Geometry check sheet. Reference: the model listing, model coordinates, mm. Face numbers are marked on the shaded views. A direction names the side the tool comes from. Coordinates: 2 decimals unless noted, no trailing zeros. Order: outer loops, then holes, each group sorted by start corner. A loop starts at its lowest first (then second) coordinate and runs counter-clockwise, first axis right, second up.
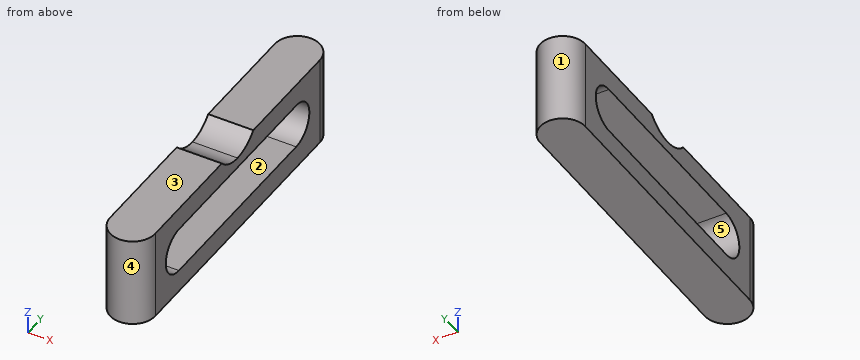
```python
from build123d import *

# Parameters (mm, degrees)
F1_DEPTH = 25.4
F3_DEPTH = 25.4
F5_DEPTH = 25.4


with BuildPart() as f1:
    # F0 (on Top) → F1 (new body)
    with BuildSketch(Plane.XY):
        with BuildLine():
            Line((-34.662835, 32.987532), (-34.662835, -46.569009))
            ThreePointArc((-34.662835, -46.569009), (-28.312835, -52.919009), (-21.962835, -46.569009))
            Line((-21.962835, -46.569009), (-21.962835, 32.987532))
            ThreePointArc((-21.962835, 32.987532), (-28.312835, 39.337532), (-34.662835, 32.987532))
        make_face()
    extrude(amount=F1_DEPTH)

    # F2 (on face) → F3 (cut)
    with BuildSketch(Plane.YZ.offset(-21.962835)):
        with BuildLine():
            Line((21.557532, 19.05), (-35.139009, 19.05))
            ThreePointArc((-35.139009, 19.05), (-41.489009, 12.7), (-35.139009, 6.35))
            Line((-35.139009, 6.35), (21.557532, 6.35))
            ThreePointArc((21.557532, 6.35), (27.907532, 12.7), (21.557532, 19.05))
        make_face()
    extrude(amount=-F3_DEPTH, mode=Mode.SUBTRACT)

    # F4 (on face) → F5 (cut)
    with BuildSketch(Plane.YZ.offset(-21.962835)):
        with BuildLine():
            Line((0.829262, 25.4), (-6.790738, 25.4))
            Line((-6.790738, 25.4), (-6.790738, 21.960208))
            ThreePointArc((-6.790738, 21.960208), (-2.61053, 22.86), (0.829262, 25.4))
        make_face()
        with BuildLine():
            Line((-6.790738, 21.960208), (-6.790738, 25.4))
            Line((-6.790738, 25.4), (-14.410738, 25.4))
            ThreePointArc((-14.410738, 25.4), (-10.970946, 22.86), (-6.790738, 21.960208))
        make_face()
    extrude(amount=-F5_DEPTH, mode=Mode.SUBTRACT)


solid = f1.part
```
Item 1: Depth check by flat-ended pin: P1, Ø2, axis at x = -30.5, z = 4, coming from the +Y side; P2, Ø1, axis at x = -23.5, z = 3, coming from the +Y side. Enter the tip coordinate at first touch or a pass-through.
Item 2: Tool access check on the marked faces 4 and 5. Record the directions out of +Z, -Z, +X, -X, +Y, -Y that give a thin tool (end or side, any length) a straight path to the whole face; none if there is none.
Item 3: Release check for a two-part mould opening along Y. For the marked faces 1, 2 and 3 record: pulls with the +Y half, pulls with the -Y half, needs draft (parallel to the pull), parting line crosses it, or undercut.
Item 4: Sectioned sample at D-D (z = 2.5). Record the cut outline in (x, y).
Item 5: Thickness scan on line 1 along Z through (x, y) = (-33.25, -19.5); line 2 along Y through (x, z) = (-32, 14.5); line 3 along Z through (x, y) = (-22.25, 24). Record the ranges inside material, lowest first.
Item 6: Sectioned sample at A-A (y = 20.5). Record the cut outline in (x, z), and give its area (3 significant figures).
Item 7: Sectioned sample at B-B (z = 12.7). Record the cut outline in (x, y).
Item 8: Sectioned sample at C-C (x = -28). Record the cut outline in (y, z).
Geometry check:
1. P1: stops at y = 39.23
1. P2: stops at y = 37.65
2. face 4: +Z, -Z, -Y
2. face 5: +X, -X
3. face 1: pulls with the +Y half
3. face 2: undercut
3. face 3: needs draft
4. outline: (-34.66, -46.57) arc R6.35 ccw to (-21.96, -46.57) - (-21.96, 32.99) arc R6.35 ccw to (-34.66, 32.99) - close
5. line 1: z = 0 to 6.35, 19.05 to 25.4
5. line 2: y = -51.74 to -41.23, 27.65 to 38.16
5. line 3: z = 0 to 6.84, 18.56 to 25.4
6. outline: (-34.66, 0) - (-21.96, 0) - (-21.96, 6.35) - (-34.66, 6.35) - close; (-34.66, 19.05) - (-21.96, 19.05) - (-21.96, 25.4) - (-34.66, 25.4) - close
6. area: 161 mm2
7. outline: (-34.66, -46.57) arc R6.35 ccw to (-21.96, -46.57) - (-21.96, -41.49) - (-34.66, -41.49) - close; (-34.66, 27.91) - (-21.96, 27.91) - (-21.96, 32.99) arc R6.35 ccw to (-34.66, 32.99) - close
8. outline: (-52.91, 0) - (39.33, 0) - (39.33, 25.4) - (0.83, 25.4) arc R10.16 cw to (-6.79, 21.96) arc R10.16 cw to (-14.41, 25.4) - (-52.91, 25.4) - close; hole (-35.14, 6.35) - (21.56, 6.35) arc R6.35 ccw to (21.56, 19.05) - (-35.14, 19.05) arc R6.35 ccw to start
